Input: part model. Units: mm. Frame: model coordinates. Coordinates: 2 decimals unless noted, no trailing zeros. Order: outer loops, then holes, each group sorted by start corner. A loop starts at its lowest first (then second) coordinate and runs counter-clockwise, first axis right, second up. Notation, with made-up numbers: M -14,58.25 L 13,58.25 A24 cw 13,83.25 Z; hole C -21.5,-1 d11. An arc over 180 degrees is marked long. One line per item, written item: value.
```python
from build123d import *

# Parameters (mm, degrees)
BOSS_EXTRUDE1_DEPTH                             = 186.947944
CUT_EXTRUDE1_DEPTH                              = 202.219677631
CUT_EXTRUDE2_DEPTH                              = 119.891891944
CSK_FOR_M3_FLAT_HEAD_MACHINE_SCREW1_D           = 3.5
CSK_FOR_M3_FLAT_HEAD_MACHINE_SCREW1_DEPTH       = 5
CSK_FOR_M3_FLAT_HEAD_MACHINE_SCREW1_CSINK_D     = 6.3
CSK_FOR_M3_FLAT_HEAD_MACHINE_SCREW1_CSINK_ANGLE = 90
CUT_EXTRUDE3_REACH                              = 142.174
SKETCH7_W                                       = 15.2
SKETCH7_H                                       = 7
SKETCH7_H_2                                     = 1


with BuildPart() as part:
    # Sketch2 → Boss-Extrude1 (new body)
    with BuildSketch(Plane(origin=(0, 0, 0), x_dir=(0, 0, -1), z_dir=(1, 0, 0))):
        Polygon((0, 0), (-2.3622, 0), (45.480481789, 57.016687901), (47.842681789, 57.016687901), align=None)
    extrude(amount=BOSS_EXTRUDE1_DEPTH)

    # Sketch3 → Cut-Extrude1 (cut, through all)
    with BuildSketch(Plane.ZY):
        Polygon((-4.105707607, 4.89299179), (-4.105707607, 7.708152127), (2.3622, 0), (0, 0), align=None)
    extrude(amount=-CUT_EXTRUDE1_DEPTH, mode=Mode.SUBTRACT)

    # Sketch4 → Cut-Extrude2 (cut, through all)
    with BuildSketch(Plane(origin=(93.496468894, -1.981357522, -4.105707607), x_dir=(-1, 0, 0), z_dir=(0, 0, -1))):
        Polygon((93.496468894, 58.998045423), (74.524995009, 58.998045423), (93.496468894, 6.874349312), align=None)
        Polygon((-93.451475106, 6.874349312), (-93.451475106, 58.998045423), (-74.480001222, 58.998045423), align=None)
    extrude(amount=CUT_EXTRUDE2_DEPTH, mode=Mode.SUBTRACT)

    # CSK for M3 Flat Head Machine Screw1
    with Locations(Plane(origin=(0, 1.163156437, 1.386195863), x_dir=(1, 0, 0), z_dir=(0, 0.6427876096865435, 0.7660444431189745))):
        with Locations((31.377677493, 46.65493708), (31.377677493, 32.145498062)):
            csk_for_m3_flat_head_machine_screw1 = CounterSinkHole(CSK_FOR_M3_FLAT_HEAD_MACHINE_SCREW1_D / 2, CSK_FOR_M3_FLAT_HEAD_MACHINE_SCREW1_CSINK_D / 2, depth=CSK_FOR_M3_FLAT_HEAD_MACHINE_SCREW1_DEPTH, counter_sink_angle=CSK_FOR_M3_FLAT_HEAD_MACHINE_SCREW1_CSINK_ANGLE)

    # Mirror1: CSK for M3 Flat Head Machine Screw1 across plane
    add(csk_for_m3_flat_head_machine_screw1.mirror(Plane(origin=(93.473972, 0, 0), x_dir=(0, 0, 1), z_dir=(1, 0, 0))), mode=Mode.SUBTRACT)

    # Cut-Extrude3: up to this plane
    cut_extrude3_end = Plane(origin=(186.947944, 0, 2.3622), z_dir=(0, -0.6427876096865434, -0.7660444431189748))
    # Sketch7 → Cut-Extrude3 (cut, up to the surface)
    with BuildSketch(Plane(origin=(112.633038957, 0, -65.028715361), x_dir=(0.4999999999999981, -1.9080601945838373e-15, 0.8660254037844397), z_dir=(-0.8660254037844397, 3.3048572009189827e-15, 0.4999999999999981)), mode=Mode.PRIVATE) as cut_extrude3_sk1:
        with Locations((53.60637797, 8.418642478)):
            Rectangle(SKETCH7_W, SKETCH7_H)
    cut_extrude3_tool1 = split(extrude(cut_extrude3_sk1.sketch, amount=CUT_EXTRUDE3_REACH, mode=Mode.PRIVATE), bisect_by=cut_extrude3_end, keep=Keep.BOTH, mode=Mode.PRIVATE)
    # Sketch7 → Cut-Extrude3 (cut, up to the surface)
    with BuildSketch(Plane(origin=(112.633038957, 0, -65.028715361), x_dir=(0.4999999999999981, -1.9080601945838373e-15, 0.8660254037844397), z_dir=(-0.8660254037844397, 3.3048572009189827e-15, 0.4999999999999981)), mode=Mode.PRIVATE) as cut_extrude3_sk2:
        with Locations((53.60637797, 4.418642478)):
            Rectangle(SKETCH7_W, SKETCH7_H_2)
    cut_extrude3_tool2 = split(extrude(cut_extrude3_sk2.sketch, amount=CUT_EXTRUDE3_REACH, mode=Mode.PRIVATE), bisect_by=cut_extrude3_end, keep=Keep.BOTH, mode=Mode.PRIVATE)
    cut_extrude3 = cut_extrude3_tool1.solids().sort_by_distance((139.436228, 8.418642, -18.60423))[0] + cut_extrude3_tool2.solids().sort_by_distance((139.436228, 4.418642, -18.60423))[0]
    add(cut_extrude3, mode=Mode.SUBTRACT)

    # Mirror2: Cut-Extrude3 across plane
    add(cut_extrude3.mirror(Plane(origin=(93.473972, 0, 0), x_dir=(0, 0, 1), z_dir=(1, 0, 0))), mode=Mode.SUBTRACT)


solid = part.part
```
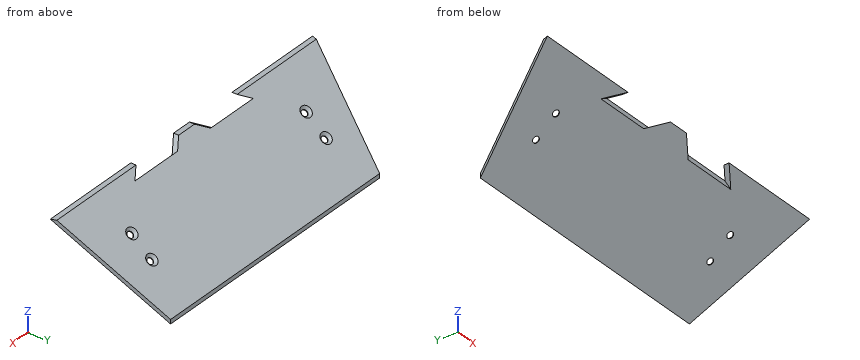
(1) Cut plane A-A on x = 112. Output: boundary loops of the cut face in (y, z), plus the area to 3 significant figures.
Data:
outline: M 11.92,-10 L 57.02,-47.84 L 57.02,-45.48 L 11.92,-7.64 Z
area: 107 mm2
(2) First-contact query: pin 1 (1.9 mm diameter, centred on x = 70, z = -9, fed in from -Y); pin 2 (2 mm diameter, centred on x = 108, y = 45.5, fed in from -Z); pin 3 (3 mm diameter, centred on x = 89, y = 29, fed in from +Z). Flat tips, straight axial feed; report the tip coordinate or a pass-through.
Data:
pin 1: stops at y = 11.92
pin 2: stops at z = -39.02
pin 3: stops at z = -20.71
(3) Cut plane B-B on z = -13. Output: boundary loops of the cut face in (x, y), plus the area to 3 significant figures.
Data:
outline: M 3.86,15.49 L 183.09,15.49 L 182.07,18.31 L 4.88,18.31 Z
area: 502 mm2
(4) Ray query, line 1 (Z direction, x = 77, y = 36.5); line 2 (Z direction, x = 171.5, y = 12); line 3 (Y direction, x = 68.5, z = -24). Return the intervals inside material, ascending. Write a range as from..to.
Data:
line 1: z = -30.63..-28.26
line 2: z = -10.07..-7.71
line 3: y = 28.6..31.42
